The model under review builds one solid part; all positions refer to its coordinate system, in mm. Face numbers are marked on the shaded views. Round coordinates to 2 decimals unless told otherwise and drop trailing zeros. Loops run counter-clockwise (first coordinate to the right, second up) from the corner with the lowest first, then second, coordinate; pieces in that order, holes last. Notation, with made-up numbers: M 71,66 L 127,66 A5 ccw 127,73 Z; hole C 58.5,-5.75 d7. An arc over 180 degrees is marked long. Use a Markdown table: item, result. Add a question column.
```python
from build123d import *

# Parameters (mm, degrees)
F0_R      = 20
F1_DEPTH  = 10
F2_R      = 17
F3_DEPTH  = 1.4
F3_FACE_R = 17
F5_R      = 16
F7_R      = 17
F8_DEPTH  = 7.1
F9_SIZE   = 1


with BuildPart() as f1:
    # F0 (on Top) → F1 (new body)
    with BuildSketch(Plane.XY):
        Circle(F0_R)
    extrude(amount=F1_DEPTH)

    # F2 (on face) → F3 (cut)
    with BuildSketch(Plane.XY.offset(10)):
        Circle(F2_R)
    extrude(amount=-F3_DEPTH, mode=Mode.SUBTRACT)

    # F3_face (on face) → F6 section 0
    with BuildSketch(Plane.XY.offset(8.6)):
        Circle(F3_FACE_R)
    # F5 (on offset) → F6 section 1
    with BuildSketch(Plane.XY.offset(7.1)):
        Circle(F5_R)
    loft(mode=Mode.SUBTRACT)

    # F7 (on face) → F8 (cut, through all)
    with BuildSketch(Plane(origin=(0, 0, 0), x_dir=(1, 0, 0), z_dir=(0, 0, -1))):
        Circle(F7_R)
    extrude(amount=-F8_DEPTH, mode=Mode.SUBTRACT)

    # F9
    f9_edges = [f1.edges().sort_by_distance(p)[0] for p in [
        (-20, 0, 10),
    ]]
    chamfer(f9_edges, length=F9_SIZE)


solid = f1.part
```
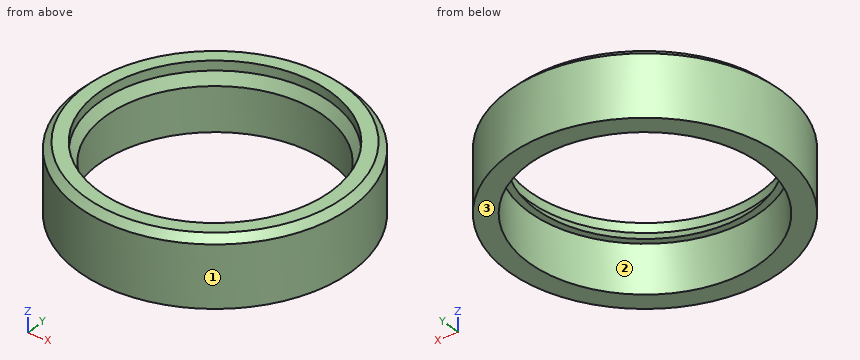
(1) To check wall thickness, follow probe 1 along Y at (x, z) = (0, 4); probe 2 along Y at (x, z) = (6.5, 9.5); probe 3 along X at (y, z) = (12, 3.75). State the ranges of each line that lie inside material, in increasing order.
(2) Draft analysis for pull direction X (two halves, no side actions). For the marked faces 1, 2 and 3, state which applies: released by +X, released by -X, zero draft, split by the parting line, or undercut.
(3) Consider section A-A, the plane x = 0. Give the boundary of the cut face in (y, z), then the cut area to 3 significant figures.
(4) Insertion check: pin 1 Ø5 at (x, z) = (2, 7.5) entering from -Y; pin 2 Ø2 at (y, z) = (14.5, 2) entering from -X; pin 3 Ø5 at (y, z) = (-11, 8) entering from +X; pin 4 Ø10 at (x, y) = (-7, -5.5) entering from -Z. Each pin has a flat end and moves straight along its axis. Give the tip position at first contact, or say it passes through.
(5) Consider section B-B, the plane z = 5.75. Give the boundary of the cut face in (x, y).
Found:
| question | item | result |
|---|---|---|
| 1 | probe 1 | y = -20 to -17, 17 to 20 |
| 1 | probe 2 | y = -18.38 to -15.71, 15.71 to 18.38 |
| 1 | probe 3 | x = -16 to -12.04, 12.04 to 16 |
| 2 | face 1 | split by the parting line |
| 2 | face 2 | undercut |
| 2 | face 3 | zero draft |
| 3 | outline | M -20,0 L -17,0 L -17,7.1 L -16,7.1 L -17,8.6 L -17,10 L -19,10 L -20,9 Z; M 16,7.1 L 17,7.1 L 17,0 L 20,0 L 20,9 L 19,10 L 17,10 L 17,8.6 Z |
| 3 | area | 60.5 mm^2 |
| 4 | pin 1 | stops at y = -20 |
| 4 | pin 2 | stops at x = -14.76 |
| 4 | pin 3 | stops at x = 18.1 |
| 4 | pin 4 | passes through |
| 5 | outline | C 0,0 d40; hole C 0,0 d34 |
